Read the model definition and answer for the solid it produces. Units are mm, in the model's axes. Face numbers are marked on the shaded views. A direction names the side the tool comes from. Give positions to 0.01 mm unless a question says otherwise; leave off trailing zeros. Write each loop counter-clockwise with the first axis right and the second up, starting at its lowest first coordinate (ties: lowest second). Pieces come first, ordered by that corner, then holes. Notation, with made-up numbers: M -14,-18.75 L 29,-18.75 A8 ccw 29,-7.75 Z; hole C -25,62.25 d4. An arc over 180 degrees is marked long. Put each result on its own line as item: value.
from build123d import *

# Parameters (mm, degrees)
SKETCH_1_R          = 1.7
SKETCH_1_R_2        = 5.4
EXTRUDE_1_DEPTH     = 10
EXTRUDE_START       = 10
EXTRUDE_2_DEPTH     = 10
CUT_EXTRUDE_START   = -10
CUT_EXTRUDE_1_DEPTH = 2
EXTRUDE_START_2     = 20
EXTRUDE_3_DEPTH     = 36
EXTRUDE_4_DEPTH     = 3.5
EXTRUDE_START_3     = 52
EXTRUDE_5_DEPTH     = 4
CUT_EXTRUDE_2_REACH = 69.936
SKETCH_7_R          = 1.7
SKETCH_7_W          = 2.5
SKETCH_7_H          = 4.5
SKETCH_8_W          = 26
SKETCH_8_H          = 10
CUT_EXTRUDE_3_DEPTH = 67.874883177
SKETCH_9_W          = 2.5
SKETCH_9_H          = 4.5
EXTRUDE_10_DEPTH    = 3
FILLET_1_R          = 2
CHAMFER_3_SIZE      = 2.5
CHAMFER_3_SIZE2     = 2


with BuildPart() as part:
    # 草图1 → 凸台-拉伸1 (new body)
    with BuildSketch(Plane.XY):
        with BuildLine():
            Line((-17, -7.5), (-17, -11))
            Line((-17, -11), (0, -11))
            ThreePointArc((0, -11), (7.778174593, -7.778174593), (11, 0))
            Line((11, 0), (11, 23.5))
            Line((11, 23.5), (-17, 23.5))
            Line((-17, 23.5), (-17, 7.5))
            ThreePointArc((-17, 7.5), (-9.5, 0), (-17, -7.5))
        make_face()
        with Locations((-5.656854249, -5.656854249)):
            Circle(SKETCH_1_R, mode=Mode.SUBTRACT)
        with Locations((5.656854249, -5.656854249)):
            Circle(SKETCH_1_R, mode=Mode.SUBTRACT)
        Circle(SKETCH_1_R_2, mode=Mode.SUBTRACT)
        with Locations((-5.656854249, 5.656854249)):
            Circle(SKETCH_1_R, mode=Mode.SUBTRACT)
        with Locations((5.656854249, 5.656854249)):
            Circle(SKETCH_1_R, mode=Mode.SUBTRACT)
    extrude(amount=EXTRUDE_1_DEPTH)

    # 草图1<6> → 凸台-拉伸2 (add)
    with BuildSketch(Plane.XY.offset(EXTRUDE_START)):
        with BuildLine():
            Line((11, 8.456854249), (11, 23.5))
            Line((11, 23.5), (-17, 23.5))
            Line((-17, 23.5), (-17, 7.5))
            ThreePointArc((-17, 7.5), (-9.5, 0), (-17, -7.5))
            Line((-17, -7.5), (-17, -11))
            ThreePointArc((-17, -11), (-8.462447466, -5.036106671), (-8.643737412, 5.376624039))
            ThreePointArc((-8.643737412, 5.376624039), (-7.46899014, 8.047704206), (-4.579821288, 8.456854249))
            Line((-4.579821288, 8.456854249), (11, 8.456854249))
        make_face()
    extrude(amount=EXTRUDE_2_DEPTH)

    # 草图3 → 切除-拉伸1 (cut)
    with BuildSketch(Plane(origin=(0, 0, 0), x_dir=(-1, 0, 0), z_dir=(0, 0, -1)).offset(CUT_EXTRUDE_START)):
        Polygon((7.919595949, 3.39411255), (8.747816894, 6.485075194), (6.485075194, 8.747816894), (3.39411255, 7.919595949), (2.565891605, 4.828633305), (4.828633305, 2.565891605), align=None)
        Polygon((-2.565891605, 4.828633305), (-3.39411255, 7.919595949), (-6.485075194, 8.747816894), (-8.747816894, 6.485075194), (-7.919595949, 3.39411255), (-4.828633305, 2.565891605), align=None)
        Polygon((-3.39411255, -7.919595949), (-2.565891605, -4.828633305), (-4.828633305, -2.565891605), (-7.919595949, -3.39411255), (-8.747816894, -6.485075194), (-6.485075194, -8.747816894), align=None)
        Polygon((2.565891605, -4.828633305), (3.39411255, -7.919595949), (6.485075194, -8.747816894), (8.747816894, -6.485075194), (7.919595949, -3.39411255), (4.828633305, -2.565891605), align=None)
    extrude(amount=CUT_EXTRUDE_1_DEPTH, mode=Mode.SUBTRACT)

    # 草图1<7> → 凸台-拉伸3 (add)
    with BuildSketch(Plane.XY.offset(EXTRUDE_START_2)):
        with BuildLine():
            Line((11, 8.456854249), (11, 23.5))
            Line((11, 23.5), (-17, 23.5))
            Line((-17, 23.5), (-17, 7.5))
            ThreePointArc((-17, 7.5), (-9.5, 0), (-17, -7.5))
            Line((-17, -7.5), (-17, -11))
            ThreePointArc((-17, -11), (-8.462447466, -5.036106671), (-8.643737412, 5.376624039))
            ThreePointArc((-8.643737412, 5.376624039), (-7.46899014, 8.047704206), (-4.579821288, 8.456854249))
            Line((-4.579821288, 8.456854249), (11, 8.456854249))
        make_face()
    extrude(amount=EXTRUDE_3_DEPTH)

    # 草图1<8> → 凸台-拉伸4 (add)
    with BuildSketch(Plane.XY):
        with BuildLine():
            Line((-17, -5), (-17, -7.5))
            ThreePointArc((-17, -7.5), (-9.5, 0), (-17, 7.5))
            Line((-17, 7.5), (-17, 5))
            ThreePointArc((-17, 5), (-12, 0), (-17, -5))
        make_face()
    extrude(amount=EXTRUDE_4_DEPTH)

    # 草图1<9> → 凸台-拉伸5 (add)
    with BuildSketch(Plane.XY.offset(EXTRUDE_START_3)):
        with BuildLine():
            Line((-17, -5), (-17, -7.5))
            ThreePointArc((-17, -7.5), (-9.5, 0), (-17, 7.5))
            Line((-17, 7.5), (-17, 5))
            ThreePointArc((-17, 5), (-12, 0), (-17, -5))
        make_face()
    extrude(amount=EXTRUDE_5_DEPTH)

    # 草图7 → 切除-拉伸2 (cut, up to next)
    with BuildSketch(Plane(origin=(0, 23.5, 0), x_dir=(1, 0, 0), z_dir=(0, 1, 0)), mode=Mode.PRIVATE) as cut_extrude_2_sk1:
        with Locations(Location((-2.879821288, -28, 0), (0, 0, 180))):
            Circle(SKETCH_7_R)
    cut_extrude_2_tool1 = extrude(cut_extrude_2_sk1.sketch, amount=-CUT_EXTRUDE_2_REACH, mode=Mode.PRIVATE) & part.part
    # 草图7 → 切除-拉伸2 (cut, up to next)
    with BuildSketch(Plane(origin=(0, 23.5, 0), x_dir=(1, 0, 0), z_dir=(0, 1, 0)), mode=Mode.PRIVATE) as cut_extrude_2_sk2:
        with Locations(Location((-2.879821288, -52, 0), (0, 0, 180))):
            Circle(SKETCH_7_R)
    cut_extrude_2_tool2 = extrude(cut_extrude_2_sk2.sketch, amount=-CUT_EXTRUDE_2_REACH, mode=Mode.PRIVATE) & part.part
    # 草图7 → 切除-拉伸2 (cut, up to next)
    with BuildSketch(Plane(origin=(0, 23.5, 0), x_dir=(1, 0, 0), z_dir=(0, 1, 0)), mode=Mode.PRIVATE) as cut_extrude_2_sk3:
        with Locations((-7.393737412, -38.75)):
            Rectangle(SKETCH_7_W, SKETCH_7_H)
    cut_extrude_2_tool3 = extrude(cut_extrude_2_sk3.sketch, amount=-CUT_EXTRUDE_2_REACH, mode=Mode.PRIVATE) & part.part
    # 草图7 → 切除-拉伸2 (cut, up to next)
    with BuildSketch(Plane(origin=(0, 23.5, 0), x_dir=(1, 0, 0), z_dir=(0, 1, 0)), mode=Mode.PRIVATE) as cut_extrude_2_sk4:
        with Locations((-7.393737412, -17.25)):
            Rectangle(SKETCH_7_W, SKETCH_7_H)
    cut_extrude_2_tool4 = extrude(cut_extrude_2_sk4.sketch, amount=-CUT_EXTRUDE_2_REACH, mode=Mode.PRIVATE) & part.part
    add(cut_extrude_2_tool1.solids().sort_by_distance((-2.879821, 23.5, 28))[0], mode=Mode.SUBTRACT)
    add(cut_extrude_2_tool2.solids().sort_by_distance((-2.879821, 23.5, 52))[0], mode=Mode.SUBTRACT)
    add(cut_extrude_2_tool3.solids().sort_by_distance((-7.393737, 23.5, 38.75))[0], mode=Mode.SUBTRACT)
    add(cut_extrude_2_tool4.solids().sort_by_distance((-7.393737, 23.5, 17.25))[0], mode=Mode.SUBTRACT)

    # 草图8 → 切除-拉伸3 (cut, through all)
    with BuildSketch(Plane(origin=(11, 0, 0), x_dir=(0, 0, -1), z_dir=(1, 0, 0))):
        with Locations((18, 15.5)):
            Rectangle(SKETCH_8_W, SKETCH_8_H)
        with BuildLine():
            ThreePointArc((-46, 19.7), (-48.787471973, 18.641655614), (-50.170131892, 16))
            ThreePointArc((-50.170131892, 16), (-50.2, 15.5), (-50.170131892, 15))
            ThreePointArc((-50.170131892, 15), (-48.787471973, 12.358344386), (-46, 11.3))
            Line((-46, 11.3), (-46, 19.7))
        make_face()
        with BuildLine():
            ThreePointArc((-41.8, 15.5), (-43.030151519, 18.469848481), (-46, 19.7))
            Line((-46, 19.7), (-46, 11.3))
            ThreePointArc((-46, 11.3), (-43.030151519, 12.530151519), (-41.8, 15.5))
        make_face()
        with BuildLine():
            ThreePointArc((-10, 11.3), (-7.212528027, 12.358344386), (-5.829868108, 15))
            ThreePointArc((-5.829868108, 15), (-5.807473676, 15.249554345), (-5.8, 15.5))
            ThreePointArc((-5.8, 15.5), (-5.807473676, 15.750445655), (-5.829868108, 16))
            ThreePointArc((-5.829868108, 16), (-7.212528027, 18.641655614), (-10, 19.7))
            Line((-10, 19.7), (-10, 11.3))
        make_face()
        with BuildLine():
            ThreePointArc((-10, 19.7), (-14.2, 15.5), (-10, 11.3))
            Line((-10, 11.3), (-10, 19.7))
        make_face()
        with BuildLine():
            Line((-50.170131892, 16), (-56, 16))
            Line((-56, 16), (-56, 15))
            Line((-56, 15), (-50.170131892, 15))
            ThreePointArc((-50.170131892, 15), (-50.2, 15.5), (-50.170131892, 16))
        make_face()
        with BuildLine():
            ThreePointArc((-5.8, 15.5), (-5.807473676, 15.249554345), (-5.829868108, 15))
            Line((-5.829868108, 15), (0, 15))
            Line((0, 15), (0, 16))
            Line((0, 16), (-5.829868108, 16))
            ThreePointArc((-5.829868108, 16), (-5.807473676, 15.750445655), (-5.8, 15.5))
        make_face()
        Polygon((-41, 10.5), (-28, 15.5), (-41, 20.5), align=None)
        Polygon((-28, 15.5), (-15, 20.5), (-41, 20.5), align=None)
        Polygon((-15, 10.5), (-15, 20.5), (-28, 15.5), align=None)
        Polygon((-15, 10.5), (-28, 15.5), (-41, 10.5), align=None)
    extrude(amount=-CUT_EXTRUDE_3_DEPTH, mode=Mode.SUBTRACT)

    # 草图9 → 凸台-拉伸10 (add)
    with BuildSketch(Plane(origin=(0, 23.5, 0), x_dir=(1, 0, 0), z_dir=(0, 1, 0))):
        with Locations((-7.393737412, -17.25)):
            Rectangle(SKETCH_9_W, SKETCH_9_H)
        with Locations((-7.393737412, -38.75)):
            Rectangle(SKETCH_9_W, SKETCH_9_H)
    extrude(amount=-EXTRUDE_10_DEPTH)

    # 圆角1
    fillet_1_edges = [part.edges().sort_by_distance(p)[0] for p in [
        (-8.643737412, 10.5, 38.75),
        (-8.643737412, 10.5, 17.25),
    ]]
    fillet(fillet_1_edges, radius=FILLET_1_R)

    # 倒角3
    chamfer_3_edges = [part.edges().sort_by_distance(p)[0] for p in [
        (-12, 0, 52),
    ]]
    chamfer_3_side = [part.faces().sort_by_distance(p)[0] for p in [
        (-12, 0, 54),
    ]]
    chamfer(chamfer_3_edges, length=CHAMFER_3_SIZE, length2=CHAMFER_3_SIZE2, reference=chamfer_3_side[0])


solid = part.part
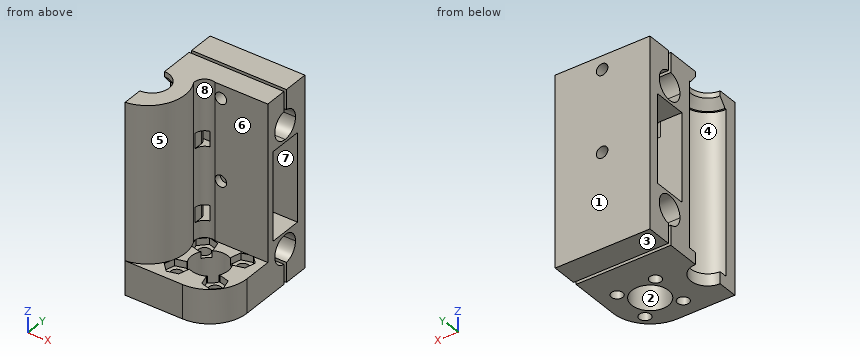
(1) Section A-A on z = 38 is taken. Determine the outline of the cut face in (x, y), and give its area (3 significant figures).
Result:
outline: M -17,-11 A11.08 ccw -8.64,5.38 A3 cw -8.64,5.94 L -8.64,8.5 A2 ccw -10.64,10.5 L -17,10.5 L -17,7.5 A7.5 cw -17,-7.5 Z; M -17,20.5 L 11,20.5 L 11,23.5 L -17,23.5 Z; M -6.14,8.62 A3 cw -4.58,8.46 L 11,8.46 L 11,10.5 L -6.14,10.5 Z
area: 204 mm²
(2) Section C-C on x = -14.5 is taken. Give the number of separate pieces and of enclosed holes in the cut face, and give its area (3 significant figures).
Result:
separate pieces: 2
enclosed holes: 1
area: 765 mm²
(3) Section B-B on z = 22 is taken. Determine the outline of the cut face in (x, y), and give its area (3 significant figures).
Result:
outline: M -17,-11 A11.08 ccw -8.64,5.38 A3 cw -4.58,8.46 L 11,8.46 L 11,10.5 L -17,10.5 L -17,7.5 A7.5 cw -17,-7.5 Z; M -17,20.5 L 11,20.5 L 11,23.5 L -17,23.5 Z
area: 211 mm²
(4) Given pin 1 Ø4 at (x, z) = (-14, 19.5) entering from -Y; pin 2 Ø5 at (x, y) = (-5.5, -5.5) entering from +Z; pin 3 Ø4.5 at (x, z) = (-2.88, 52) entering from -Y; pin 4 Ø4 at (y, z) = (13, 27) entering from -X, each flat-ended and moving along its own axis, determine where each tip first touches the part or whether it passes through.
Result:
pin 1: stops at y = -10.83
pin 2: stops at z = 8
pin 3: stops at y = 8.46
pin 4: passes through
(5) Which of the six approach directions +Z, -Z, +X, -X, +Y, -Y give full straight-line access (tool end or side, diameter ignored) to the marked faces 4, 5, 6, 7 and 8?
Result:
face 4: -X
face 5: +Z, +X
face 6: +Z, +X, -Y
face 7: +X, -X
face 8: +Z
(6) For a pull along Y with two mould halves and no side action, classify the marked faces 1, 2 and 3 as +Y half, -Y half, draft (parallel to the pull), parting line (faces both ways), or undercut.
Result:
face 1: +Y half
face 2: undercut
face 3: draft
(7) Straight lines are drawn through the part: line 1 along Y through (x, z) = (0, 2.5); line 2 along Y through (x, z) = (2, 7.5); line 3 along Z through (x, y) = (0.25, 16.5). For each, find the intervals that lie inside material, in ascending order. Write a range as from..to.
Result:
line 1: y = -11..-5.4, 5.4..15, 16..23.5
line 2: y = -10.82..-5.02, 5.02..12.13, 18.87..23.5
line 3: z = 0..5.92, 14.08..15, 41..41.92, 50.08..56
